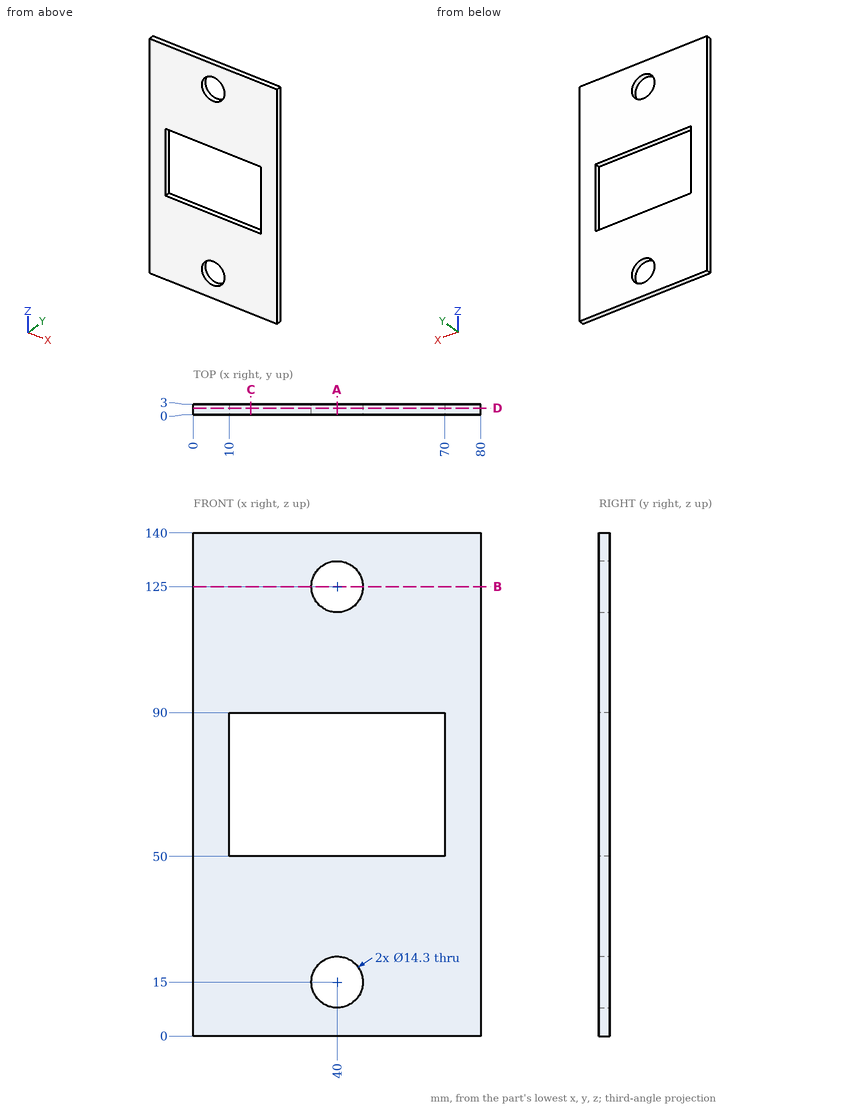
The drawing under review shows one solid part. Ordinate dimensions are in mm from its lowest x, y, z. Coordinates: 2 decimals unless noted, no trailing zeros. Write each loop counter-clockwise with the first axis right and the second up, starting at its lowest first coordinate (ties: lowest second). Pieces come first, ordered by that corner, then holes. Notation, with made-up numbers: (62, 36) - (72, 36) arc R25 ccw to (72, 61) - close; hole circle Ø1 at (14.5, 36). An arc over 180 degrees is marked (long way). Put each result on its own line as item: value.
1. Add section B-B, the plane z = 125. Give the boundary of the cut face in (x, y), then the cut area to 3 significant figures.
Values found:
outline: (0, 0) - (32.85, 0) - (32.85, 3) - (0, 3) - close; (47.15, 0) - (80, 0) - (80, 3) - (47.15, 3) - close
area: 197 mm²
2. For pin 1 (11.5 mm diameter, centred on x = 40, z = 125, fed in from -Y), flat-tipped, find the tip position at first contact; note if it passes through.
Values found:
pin 1: through
3. Add section D-D, the plane y = 1.85. Give the boundary of the cut face in (x, z), then the cut area to 3 significant figures.
Values found:
outline: (0, 0) - (80, 0) - (80, 140) - (0, 140) - close; hole (10, 50) - (70, 50) - (70, 90) - (10, 90) - close; hole circle Ø14.3 at (40, 15); hole circle Ø14.3 at (40, 125)
area: 8,480 mm²
4. Add section A-A, the plane x = 40. Give the boundary of the cut face in (y, z).
Values found:
outline: (0, 0) - (3, 0) - (3, 7.85) - (0, 7.85) - close; (0, 22.15) - (3, 22.15) - (3, 50) - (0, 50) - close; (0, 90) - (3, 90) - (3, 117.85) - (0, 117.85) - close; (0, 132.15) - (3, 132.15) - (3, 140) - (0, 140) - close
5. Add section C-C, the plane x = 16. Give the boundary of the cut face in (y, z).
Values found:
outline: (0, 0) - (3, 0) - (3, 50) - (0, 50) - close; (0, 90) - (3, 90) - (3, 140) - (0, 140) - close
6. Wall thickness on probe 1 along Z at (x, y) = (40, 0.7); probe 2 along Z at (x, y) = (25, 0.15); probe 3 along X at (y, z) = (1.95, 15): over which ranges is each line inside the solid? List them lowest first.
Values found:
probe 1: 0 to 7.85, 22.15 to 50, 90 to 117.85, 132.15 to 140
probe 2: 0 to 50, 90 to 140
probe 3: 0 to 32.85, 47.15 to 80
